Source: CAD feature listing. Evaluate the final solid. Frame: model axes, mm. Face numbers are marked on the shaded views. A direction names the side the tool comes from. Give positions to 0.01 mm unless a question says otherwise; leave off trailing zeros. Order: outer loops, then holes, each group sorted by start corner. A loop starts at its lowest first (then second) coordinate and runs counter-clockwise, first axis right, second up.
1) Access query for the marked faces 4, 5 and 6. Directions: +Z, -Z, +X, -X, +Y, -Y. A direction counts if a zero-diameter tool reaches every point of the face in a straight line with its end or side. Return the directions, or none.
2) Material intervals for line 1 (X direction, y = 1.5, z = 0.95); line 2 (X direction, y = -0.5, z = 1.4); line 3 (Z direction, x = 2.3, y = 2.25), sorted ascending.
3) Section A-A, the plane y = 2.75. Return loops of the section in (x, z).
4) First-contact query: P1, Ø1.2, axis at x = 0.5, z = 1.5, coming from the -Y side; P2, Ø2, axis at x = 0.5, y = 3, coming from the +Z side; P3, Ø0.6, axis at x = 2.5, y = 3, coming from the -Z side. Flat tips, straight axial feed; report the tip coordinate or a pass-through.
5) Section B-B, the plane x = 0.7. Return loops of the section in (y, z).
6) Draft query along X for the marked faces 1, 2 and 3. Return one class per face: released by +X, released by -X, zero draft, split by the parting line, or undercut.
7) Section C-C, the plane z = 0.4. Return loops of the section in (x, y).
```python
from build123d import *

# Parameters (mm, degrees)
BOSS_EXTRUDE1_DEPTH = 2.58
CUT_EXTRUDE1_DEPTH  = 10.5
CUT_EXTRUDE2_DEPTH  = 5.25
BOSS_EXTRUDE2_DEPTH = 0.5
SKETCH5_W           = 2.430822105
SKETCH5_H           = 5.029930807
CUT_EXTRUDE3_DEPTH  = 1
CHAMFER1_SIZE       = 0.6
CHAMFER2_SIZE       = 0.4


with BuildPart() as part:
    # Sketch1 → Boss-Extrude1 (new body)
    with BuildSketch(Plane.XY):
        with BuildLine():
            Line((-2.75, -4), (-2.75, 4.05))
            ThreePointArc((-2.75, 4.05), (-2.544974747, 4.544974747), (-2.05, 4.75))
            Line((-2.05, 4.75), (2.05, 4.75))
            ThreePointArc((2.05, 4.75), (2.544974747, 4.544974747), (2.75, 4.05))
            Line((2.75, 4.05), (2.75, -4))
            Line((2.75, -4), (2.25, -4))
            Line((2.25, -4), (2.25, 4.05))
            ThreePointArc((2.25, 4.05), (2.191421356, 4.191421356), (2.05, 4.25))
            Line((2.05, 4.25), (-2.05, 4.25))
            ThreePointArc((-2.05, 4.25), (-2.191421356, 4.191421356), (-2.25, 4.05))
            Line((-2.25, 4.05), (-2.25, -4))
            Line((-2.25, -4), (-2.75, -4))
        make_face()
    extrude(amount=BOSS_EXTRUDE1_DEPTH)

    # Sketch2 → Cut-Extrude1 (cut)
    with BuildSketch(Plane(origin=(0, 4.75, 0), x_dir=(1, 0, 0), z_dir=(0, 1, 0))):
        Polygon((-2, -0.58), (-4.099439411, -0.58), (-4.099439411, 0.833357165), (-2, 0.833357165), (-1.6, 0), align=None)
        Polygon((2, -0.58), (3.357409655, -0.58), (3.357409655, 0.833357165), (2, 0.833357165), (1.6, 0), align=None)
        with BuildLine():
            Line((-2.75, -2.58), (-2.38062097, -2.58))
            ThreePointArc((-2.38062097, -2.58), (-2.104839164, -2.497066416), (-1.920543652, -2.275777582))
            Line((-1.920543652, -2.275777582), (-1.314728174, -0.852111209))
            ThreePointArc((-1.314728174, -0.852111209), (-1.222580418, -0.741466792), (-1.084689515, -0.7))
            Line((-1.084689515, -0.7), (1.084290526, -0.7))
            ThreePointArc((1.084290526, -0.7), (1.222412736, -0.741619926), (1.314545856, -0.852621958))
            Line((1.314545856, -0.852621958), (1.915985292, -2.274756083))
            ThreePointArc((1.915985292, -2.274756083), (2.100251533, -2.496760148), (2.376495952, -2.58))
            Line((2.376495952, -2.58), (2.75, -2.58))
            Line((2.75, -2.58), (2.75, -3.056093585))
            Line((2.75, -3.056093585), (-2.75, -3.056093585))
            Line((-2.75, -3.056093585), (-2.75, -2.58))
        make_face()
    extrude(amount=-CUT_EXTRUDE1_DEPTH, mode=Mode.SUBTRACT)

    # Sketch3 → Cut-Extrude2 (cut, symmetric)
    with BuildSketch(Plane(origin=(0, 0, 0), x_dir=(0, 0, -1), z_dir=(1, 0, 0))):
        Polygon((-0.58, 0.25), (-1.08, -0.35), (-1.08, -4.396314828), (-0.130305992, -4.396314828), (-0.130305992, 0.25), align=None)
        Polygon((-2.58, 0.25), (-2.08, -0.35), (-2.08, -4.896314828), (-3.070294312, -4.896314828), (-3.070294312, 0.25), align=None)
        with BuildLine():
            Line((-1.08, 3.024565065), (-1.08, 1.024565065))
            ThreePointArc((-1.08, 1.024565065), (-1.58, 0.524565065), (-2.08, 1.024565065))
            Line((-2.08, 1.024565065), (-2.08, 3.024565065))
            ThreePointArc((-2.08, 3.024565065), (-1.58, 3.524565065), (-1.08, 3.024565065))
        make_face()
    extrude(amount=CUT_EXTRUDE2_DEPTH, both=True, mode=Mode.SUBTRACT)

    # Sketch4 → Boss-Extrude2 (add, symmetric)
    with BuildSketch(Plane(origin=(0, 0, 0), x_dir=(0, 0, -1), z_dir=(1, 0, 0))):
        with BuildLine():
            Line((-0.7, 4.25), (-1.045169213, 3.954140675))
            ThreePointArc((-1.045169213, 3.954140675), (-1.420160684, 3.782160221), (-1.829373497, 3.834512432))
            Line((-1.829373497, 3.834512432), (-2.4, 4.079724782))
            Line((-2.4, 4.079724782), (-2.202592831, 4.539105245))
            Line((-2.202592831, 4.539105245), (-1.631966328, 4.293892895))
            ThreePointArc((-1.631966328, 4.293892895), (-1.495562057, 4.276442158), (-1.3705649, 4.333768976))
            Line((-1.3705649, 4.333768976), (-0.997308957, 4.653702641))
            ThreePointArc((-0.997308957, 4.653702641), (-0.875770907, 4.725154006), (-0.736992408, 4.75))
            Line((-0.736992408, 4.75), (-0.7, 4.75))
            Line((-0.7, 4.75), (-0.7, 4.25))
        make_face()
    extrude(amount=BOSS_EXTRUDE2_DEPTH, both=True)

    # Sketch5 → Cut-Extrude3 (cut)
    with BuildSketch(Plane.ZY.offset(2.75)):
        with Locations((1.671482724, -2.864965403)):
            Rectangle(SKETCH5_W, SKETCH5_H)
    extrude(amount=-CUT_EXTRUDE3_DEPTH, mode=Mode.SUBTRACT)

    # Chamfer1
    chamfer1_edges = [part.edges().sort_by_distance(p)[0] for p in [
        (2.5, -4, 1.08),
    ]]
    chamfer(chamfer1_edges, length=CHAMFER1_SIZE)

    # Chamfer2
    chamfer2_edges = [part.edges().sort_by_distance(p)[0] for p in [
        (2.5, -4, 2.08),
    ]]
    chamfer(chamfer2_edges, length=CHAMFER2_SIZE - 0.0001)  # a hair under: the kernel refuses the full size


solid = part.part
```
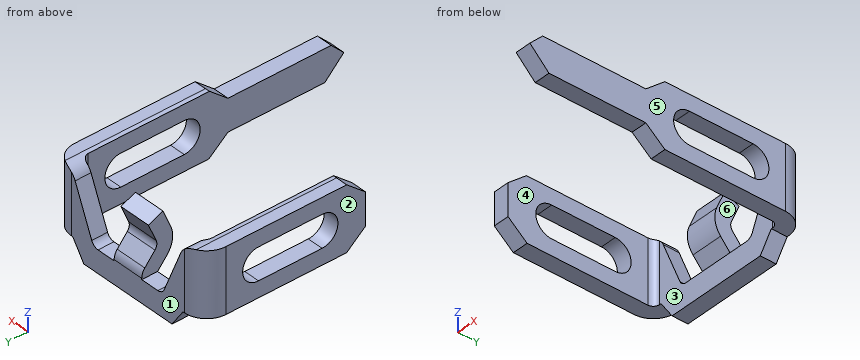
From the geometry:
1. face 4: +Z, -Z, -Y
1. face 5: +Z, -Z, +X, +Y, -Y
1. face 6: +Z, +Y, -Y
2. line 1: x = -2.75 to -2.25, 2.25 to 2.75
2. line 2: x = 2.25 to 2.75
2. line 3: z = 0.58 to 1.08, 2.08 to 2.57
3. outline: (-2.75, 0.58) - (-2.25, 0.58) - (-2.25, 1.08) - (-2.75, 1.08) - close; (-2.75, 2.08) - (-2.25, 2.08) - (-2.25, 2.56) arc R0.5 ccw to (-2.38, 2.58) - (-2.75, 2.58) - close; (2.25, 0.58) - (2.75, 0.58) - (2.75, 1.08) - (2.25, 1.08) - close; (2.25, 2.08) - (2.75, 2.08) - (2.75, 2.58) - (2.38, 2.58) arc R0.5 ccw to (2.25, 2.56) - close
4. P1: stops at y = 3.77
4. P2: stops at z = 2.21
4. P3: stops at z = 0.58
5. outline: (4.25, 0) - (4.75, 0) - (4.75, 0.7) - (4.25, 0.7) - close
6. face 1: zero draft
6. face 2: released by -X
6. face 3: undercut
7. outline: (-1.88, 4.25) - (1.88, 4.25) - (1.88, 4.75) - (-1.88, 4.75) - close
